Geometry check sheet. Reference: the model listing, model coordinates, mm. A direction names the side the tool comes from. Round coordinates to 2 decimals unless told otherwise and drop trailing zeros. Order: outer loops, then holes, each group sorted by start corner. A loop starts at its lowest first (then second) coordinate and runs counter-clockwise, first axis right, second up. Notation, with made-up numbers: (-14, 23) - (23, 23) arc R35 cw to (23, 62) - close; hole circle Ø3 at (81.5, 71.5). An arc over 180 degrees is marked (long way). Return JSON: item names as keys, results as strings. Group by question number.
Q1. Material ranges on line 1 along Y through (x, z) = (-15, 4.8); line 2 along Y through (x, z) = (1.5, 1.4); line 3 along X through (y, z) = (-12.25, 0.2), recorded low to high.
Q2. Sectioned sample at B-B, the plane z = 4.75. Record the cut outline in (x, y), then the cut area to 3 significant figures.
Q3. Gauge pin test, flat ends, axial feed: pin 1 Ø1.6 at (y, z) = (-15.5, 1.5) entering from +X; pin 2 Ø1.3 at (x, z) = (-19, 4) entering from -Y; pin 3 Ø1.3 at (x, z) = (-6.5, 2.5) entering from +Y. Record the tip position at first contact, or that the pin passes through.
Q4. Sectioned sample at A-A, the plane x = -6. Record the cut outline in (y, z), then the cut area to 3 significant figures.
Q5. Sectioned sample at C-C, the plane y = 6.75. Record the cut outline in (x, z), then the cut area to 3 significant figures.
Q6. Tool access check on faces 1 (the flat face through (-3, 8.55, 3)), 2 (the flat face through (8, -10.55, 3)), 3 (the flat face through (-14, -16, 1)). Record the directions out of +Z, -Z, +X, -X, +Y, -Y that give a thin tool (end or side, any length) a straight path to the whole face; none if there is none.
```python
from build123d import *

# Parameters (mm, degrees)
F1_DEPTH = 1
F3_DEPTH = 4.5


with BuildPart() as f1:
    # F0 (on Top) → F1 (new body)
    with BuildSketch(Plane.XY):
        Polygon((-2.55, -10.55), (25.65, -10.55), (25.65, 10.55), (-2.55, 10.55), (-25.65, 10.55), (-25.65, -10.55), (-25.65, -17.55), (-2.55, -17.55), align=None)
    extrude(amount=F1_DEPTH)

    # F2 (on face) → F3 (join)
    with BuildSketch(Plane.XY.offset(1)):
        Polygon((18.65, -10.55), (18.65, 8.55), (-25.65, 8.55), (-25.65, -15.05), (-2.55, -15.05), (-2.55, -10.55), align=None)
    extrude(amount=F3_DEPTH)


solid = f1.part
```
Reply:
{
 "1": {"line 1": "-15.05 to 8.55", "line 2": "-10.55 to 8.55", "line 3": "-25.65 to -2.55"},
 "2": {"outline": "(-25.65, -15.05) - (-2.55, -15.05) - (-2.55, -10.55) - (18.65, -10.55) - (18.65, 8.55) - (-25.65, 8.55) - close", "area": "950 mm^2"},
 "3": {"pin 1": "x = -2.55", "pin 2": "y = -15.05", "pin 3": "y = 8.55"},
 "4": {"outline": "(-17.55, 0) - (10.55, 0) - (10.55, 1) - (8.55, 1) - (8.55, 5.5) - (-15.05, 5.5) - (-15.05, 1) - (-17.55, 1) - close", "area": "134 mm^2"},
 "5": {"outline": "(-25.65, 0) - (25.65, 0) - (25.65, 1) - (18.65, 1) - (18.65, 5.5) - (-25.65, 5.5) - close", "area": "251 mm^2"},
 "6": {"face 1": "+Z, +X, -X, +Y", "face 2": "+Z, -Z, +X, -Y", "face 3": "+Z, +X, -X, -Y"}
}
